```python
from build123d import *

# Parameters (mm, degrees)
ESTRUSIONE_ESTRUSIONE1_DEPTH = 3
SCHIZZO2_R                   = 2.25
TAGLIO_ESTRUSIONE1_DEPTH     = 131.62050005


with BuildPart() as part:
    # Schizzo1 → Estrusione-Estrusione1 (new body)
    with BuildSketch(Plane.XY):
        with BuildLine():
            ThreePointArc((116.244263144, 0), (112.553023812, 29.061065786), (101.713730251, 56.276511906))
            ThreePointArc((101.713730251, 56.276511906), (93.227009104, 58.717251262), (90.786269749, 50.230530114))
            ThreePointArc((90.786269749, 50.230530114), (100.461060229, 25.938934214), (103.755736856, 0))
            ThreePointArc((103.755736856, 0), (110, -6.244263144), (116.244263144, 0))
        make_face()
    extrude(amount=ESTRUSIONE_ESTRUSIONE1_DEPTH)

    # Schizzo2 → Taglio-Estrusione1 (cut, through all)
    with BuildSketch(Plane(origin=(0, 0, 0), x_dir=(-1, 0, 0), z_dir=(0, 0, -1))):
        with Locations((-110, 0)):
            Circle(SCHIZZO2_R)
        with Locations((-96.25, 53.25352101)):
            Circle(SCHIZZO2_R)
    extrude(amount=-TAGLIO_ESTRUSIONE1_DEPTH, mode=Mode.SUBTRACT)


solid = part.part
```
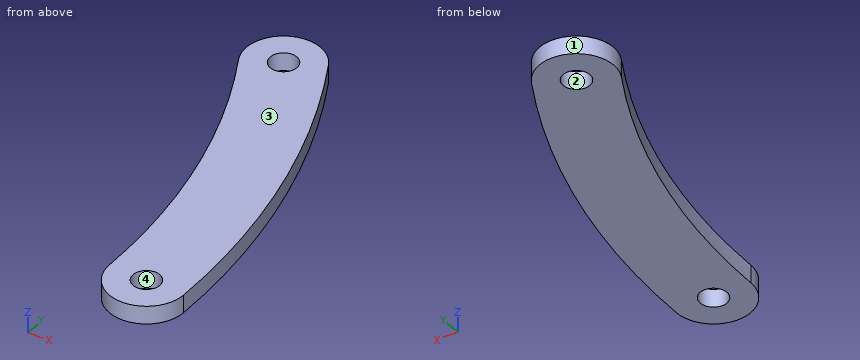
The listing builds one solid part. Answer for the finished solid, in the listing's coordinates (mm). Face numbers are marked on the shaded views. Give positions to 0.01 mm unless a question says otherwise; leave off trailing zeros. Write each loop counter-clockwise with the first axis right and the second up, starting at its lowest first coordinate (ties: lowest second). Pieces come first, ordered by that corner, then holes. Notation, with made-up numbers: (21.5, 58) - (63.5, 58) arc R28 ccw to (63.5, 79) - close; hole circle Ø10 at (-29, -34). An arc over 180 degrees is marked (long way). Use one line per item in the form item = value. Start each with the question number.
1) Find section B-B on x = 96.25. Determine the outline of the cut face in (y, z).
2) Find section A-A on y = 1.5. Determine the outline of the cut face in (x, z), plus the area to 3 significant figures.
3) Find section C-C on z = 1.4. Determine the outline of the cut face in (x, y).
4) A flat-ended cylindrical pin translates along its axis: pin 1 Ø1.5 at (y, z) = (44, 1.5) entering from -X. Find the tip coordinate at first contact, or state that the pin passes through.
5) Consider line 1 along Y through (x, z) = (108, 2.85); line 2 along X through (y, z) = (36, 1.8); line 3 along X through (y, z) = (29, 0.25). Determine where each line is inside the solid, lowest interval first. Write a range as from..to.
6) Find section D-D on y = 26. Determine the outline of the cut face in (x, z), plus the area to 3 significant figures.
7) The mould has two halves that part along Y. Classify the marked faces 1, 2, 3 and 4: pulls with the +Y half, pulls with the -Y half, needs draft (parallel to the pull), parting line crosses it, or undercut.
Geometry results:
q1.outline = (38.75, 0) - (51, 0) - (51, 3) - (38.75, 3) - close; (55.5, 0) - (59.5, 0) - (59.5, 3) - (55.5, 3) - close
q2.outline = (103.74, 0) - (108.32, 0) - (108.32, 3) - (103.74, 3) - close; (111.68, 0) - (116.23, 0) - (116.23, 3) - (111.68, 3) - close
q2.area = 27.4 mm2
q3.outline = (90.79, 50.23) arc R103.76 cw to (103.76, 0) arc R6.24 ccw to (116.24, 0) arc R116.24 ccw to (101.71, 56.28) arc R6.24 ccw to start; hole circle Ø4.5 at (96.25, 53.25); hole circle Ø4.5 at (110, 0)
q4.pin_1 = 93.61
q5.line_1 = -5.92..-1.03, 1.03..43
q5.line_2 = 97.31..110.53
q5.line_3 = 99.62..112.57
q6.outline = (100.45, 0) - (113.3, 0) - (113.3, 3) - (100.45, 3) - close
q6.area = 38.6 mm2
q7.face_1 = parting line crosses it
q7.face_2 = undercut
q7.face_3 = needs draft
q7.face_4 = undercut
